Source: CAD feature listing. Evaluate the final solid. Frame: model axes, mm. A direction names the side the tool comes from. Round coordinates to 2 decimals unless told otherwise and drop trailing zeros. Order: outer loops, then holes, each group sorted by start corner. A loop starts at its lowest first (then second) coordinate and runs counter-clockwise, first axis right, second up. Notation, with made-up numbers: (67.25, 25.5) -> (124.25, 25.5) arc R36 cw to (124.25, 59.5) -> close; hole circle Ø8 at (-32.75, 56.25). An arc over 180 degrees is marked (long way). Answer as CSV lines item,"result".
from build123d import *

# Parameters (mm, degrees)
SKETCH1_R                   = 12
BOSS_EXTRUDE1_DEPTH         = 3
TAP_DRILL_FOR_M3_TAP1_D     = 2.5
TAP_DRILL_FOR_M3_TAP1_DEPTH = 5
TAP_DRILL_FOR_M3_TAP1_TIP   = 0.751075774
TAP_DRILL_FOR_M4_TAP1_D     = 5
TAP_DRILL_FOR_M4_TAP1_DEPTH = 5
TAP_DRILL_FOR_M4_TAP1_TIP   = 1.502151548
FILLET1_R                   = 2
TAP_DRILL_FOR_M2_TAP1_D     = 1.6
TAP_DRILL_FOR_M2_TAP1_DEPTH = 5
TAP_DRILL_FOR_M2_TAP1_TIP   = 0.480688495
CUT_EXTRUDE1_DEPTH          = 10


with BuildPart() as part:
    # Sketch1 → Boss-Extrude1 (new body)
    with BuildSketch(Plane.XY):
        Polygon((18.05, -56.055), (18.05, -21.05), (21.05, -18.05), (21.05, 18.05), (18.05, 21.05), (-18.05, 21.05), (-21.05, 18.05), (-21.05, -18.05), (-18.05, -21.05), (-18.05, -56.055), align=None)
        Circle(SKETCH1_R, mode=Mode.SUBTRACT)
    extrude(amount=BOSS_EXTRUDE1_DEPTH)

    # Tap Drill for M3 Tap1
    with Locations(Plane.XY.offset(3)):
        with Locations((-15.5, 15.5), (15.5, 15.5), (-15.5, -15.5), (15.5, -15.5)):
            Hole(TAP_DRILL_FOR_M3_TAP1_D / 2, depth=TAP_DRILL_FOR_M3_TAP1_DEPTH)
            with Locations((0, 0, -(TAP_DRILL_FOR_M3_TAP1_DEPTH + TAP_DRILL_FOR_M3_TAP1_TIP / 2))):  # 118° drill point
                Cone(0, TAP_DRILL_FOR_M3_TAP1_D / 2, TAP_DRILL_FOR_M3_TAP1_TIP, mode=Mode.SUBTRACT)

    # Tap Drill for M4 Tap1
    with Locations(Plane.XY.offset(3)):
        with Locations((12, -41.055), (-12, -41.055)):
            Hole(TAP_DRILL_FOR_M4_TAP1_D / 2, depth=TAP_DRILL_FOR_M4_TAP1_DEPTH)
            with Locations((0, 0, -(TAP_DRILL_FOR_M4_TAP1_DEPTH + TAP_DRILL_FOR_M4_TAP1_TIP / 2))):  # 118° drill point
                Cone(0, TAP_DRILL_FOR_M4_TAP1_D / 2, TAP_DRILL_FOR_M4_TAP1_TIP, mode=Mode.SUBTRACT)

    # Fillet1
    fillet1_edges = [part.edges().sort_by_distance(p)[0] for p in [
        (18.05, -21.05, 1.5),
        (18.05, -56.055, 1.5),
        (-18.05, -56.055, 1.5),
        (-18.05, -21.05, 1.5),
    ]]
    fillet(fillet1_edges, radius=FILLET1_R)

    # Tap Drill for M2 Tap1
    with Locations(Plane.XY.offset(3)):
        with Locations((10.52945603, -21.86131015), (10.52945603, -28.56131015)):
            Hole(TAP_DRILL_FOR_M2_TAP1_D / 2, depth=TAP_DRILL_FOR_M2_TAP1_DEPTH)
            with Locations((0, 0, -(TAP_DRILL_FOR_M2_TAP1_DEPTH + TAP_DRILL_FOR_M2_TAP1_TIP / 2))):  # 118° drill point
                Cone(0, TAP_DRILL_FOR_M2_TAP1_D / 2, TAP_DRILL_FOR_M2_TAP1_TIP, mode=Mode.SUBTRACT)

    # Sketch8 → Cut-Extrude1 (cut)
    with BuildSketch(Plane.XY):
        with BuildLine():
            Line((0.899883871, -36.671612752), (-0.221262765, -38.266132411))
            ThreePointArc((-0.221262765, -38.266132411), (-2.432977147, -38.651660606), (-2.818505343, -36.439946223))
            Line((-2.818505343, -36.439946223), (-1.341666159, -34.339552718))
            Line((-1.341666159, -34.339552718), (-2.655433384, -32.972737792))
            ThreePointArc((-2.655433384, -32.972737792), (-2.611361373, -30.745711142), (-0.384334723, -30.789783153))
            Line((-0.384334723, -30.789783153), (0.504250938, -31.714248402))
            Line((0.504250938, -31.714248402), (1.028839157, -30.968167379))
            ThreePointArc((1.028839157, -30.968167379), (3.24055354, -30.582639184), (3.626081735, -32.794353566))
            Line((3.626081735, -32.794353566), (2.745800968, -34.046308435))
            Line((2.745800968, -34.046308435), (4.580323387, -35.954905771))
            ThreePointArc((4.580323387, -35.954905771), (4.536251377, -38.181932421), (2.309224727, -38.137860411))
            Line((2.309224727, -38.137860411), (0.899883871, -36.671612752))
        make_face()
    extrude(amount=CUT_EXTRUDE1_DEPTH, mode=Mode.SUBTRACT)


solid = part.part
1. Line query: L1, parallel to Y at x = -15.5, z = 1.2 (3 decimals); L2, parallel to X at y = -38, z = 2; L3, parallel to X at y = -41.5, z = 2.5. Output: solid intervals per line, ascending. Write a range as [from, to].
Results below:
L1,"[-56.055, -16.75], [-14.25, 14.25], [16.75, 21.05]"
L2,"[-18.05, -2.97], [-0.03, 2.18], [4.7, 18.05]"
L3,"[-18.05, -14.46], [-9.54, 9.54], [14.46, 18.05]"
2. Section query D-D on z = 1.6. Give the number of separate pieces and of enclosed holes in the cut face, and give its area (3 significant figures).
Results below:
separate pieces,"1"
enclosed holes,"10"
area,"2,450 mm2"
3. Section query B-B on y = 15.5. Return loops of the section in (x, z).
Results below:
outline,"(-21.05, 0) -> (-16.75, 0) -> (-16.75, 3) -> (-21.05, 3) -> close; (-14.25, 0) -> (14.25, 0) -> (14.25, 3) -> (-14.25, 3) -> close; (16.75, 0) -> (21.05, 0) -> (21.05, 3) -> (16.75, 3) -> close"
4. Section query C-C on x = -5. Return loops of the section in (y, z) (3 decimals), and give its area (3 significant figures).
Results below:
outline,"(-56.055, 0) -> (-10.909, 0) -> (-10.909, 3) -> (-56.055, 3) -> close; (10.909, 0) -> (21.05, 0) -> (21.05, 3) -> (10.909, 3) -> close"
area,"166 mm2"
5. Section query A-A on y = 0. Return loops of the section in (x, z).
Results below:
outline,"(-21.05, 0) -> (-12, 0) -> (-12, 3) -> (-21.05, 3) -> close; (12, 0) -> (21.05, 0) -> (21.05, 3) -> (12, 3) -> close"
6. Reachability of faces 1 (the flat face through (1.6, -37.4, 1.5)), 2 (the flat face through (18.05, -38, 1)), 3 (the flat face through (-19.5, 19.6, 1.5)) from +Z, -Z, +X, -X, +Y, -Y: full face, straight path, thin tool, end or side. Return the list, or none.
Results below:
face 1,"+Z, -Z"
face 2,"+Z, -Z, +X, -Y"
face 3,"+Z, -Z, -X, +Y"
7. Pin query (flat end, axial travel): pin 1 (2 mm diameter, centred on x = -15.5, y = 15.5, fed in from -Z). Return the tip coordinate at first contact, or that it passes through.
Results below:
pin 1,"through"
